The model under review builds one solid part; all positions refer to its coordinate system, in mm. A direction names the side the tool comes from. Coordinates: 2 decimals unless noted, no trailing zeros. Write each loop counter-clockwise with the first axis right and the second up, starting at its lowest first coordinate (ties: lowest second). Pieces come first, ordered by that corner, then holes. Notation, with made-up numbers: (5, -39.5) - (32, -39.5) arc R22 cw to (32, -21.5) - close; hole circle Ø8 at (3.5, 67.25). An arc over 180 degrees is marked (long way). Return JSON: item names as keys, results as strings. Group by question number.
(1) We need section D-D on x = -22.5. State the section outline as (y, z) points, then the cut area to 3 significant figures.
(2) To check wall thickness, follow L1, parallel to X at y = 18.75, z = 26; L2, parallel to Z at x = -27, y = 4; L3, parallel to Y at x = 6, z = 4.5. State the ranges of each line that lie inside material, in increasing order. Write a range as from..to.
(3) We need section B-B on z = -10. State the section outline as (x, y) points, then the cut area to 3 significant figures.
(4) We need section C-C on y = 5. State the section outline as (x, z) points.
(5) We need section A-A on y = 28.25. State the section outline as (x, z) points.
(6) For pin 1 Ø1.5 at (x, y) = (-38.5, 9) entering from +Z; pin 2 Ø3 at (x, z) = (19, 0) entering from +Y; pin 3 Ø1.5 at (x, y) = (-39, 7.5) entering from +Z, all flat-tipped, find the tip position at first contact; note any pin that passes through.
(7) Tool access review of faces 1 (the face through (-38.498, 12.077, -5.534)), 2 (the face through (-4, 16, -25.555)), 3 (the face through (-39.122, 14.79, -27.653)): name each direction out of +Z, -Z, +X, -X, +Y, -Y from which nothing blocks a thin tool from reaching the whole face with its end or side.
(8) Draft analysis for pull direction X (two halves, no side actions). For faces 4 (the face through (-39.977, 15, 12)), 5 (the face through (-38, 13.596, -10)), 6 (the face through (-36.38, 15.7, 47.87)), state which applies: released by +X, released by -X, zero draft, split by the parting line, or undercut.
```python
from build123d import *

# Parameters (mm, degrees)
BOSS_EXTRUDE1_DEPTH = 30
CUT_EXTRUDE1_DEPTH  = 29
CUT_EXTRUDE3_DEPTH  = 10
SKETCH6_W           = 27.115913197
SKETCH6_H           = 16.602687323
BOSS_EXTRUDE2_DEPTH = 3
SKETCH7_W           = 8.89
SKETCH7_H           = 10.922
CUT_EXTRUDE4_DEPTH  = 6350
BOSS_EXTRUDE3_START = -3
SKETCH8_W           = 8.89
SKETCH8_H           = 10.922
BOSS_EXTRUDE3_DEPTH = 3
BOSS_EXTRUDE4_START = -3
SKETCH9_W           = 8.89
SKETCH9_H           = 10.922
BOSS_EXTRUDE4_DEPTH = 3
SKETCH12_W          = 9
SKETCH12_H          = 11
CUT_EXTRUDE6_DEPTH  = 3


with BuildPart() as part:
    # Sketch2 → Boss-Extrude1 (new body)
    with BuildSketch(Plane(origin=(0, 0, 0), x_dir=(1, 0, 0), z_dir=(0, 1, 0))):
        with BuildLine():
            Line((-36.97733711, 28.555240793), (29.02266289, 28.555240793))
            ThreePointArc((29.02266289, 28.555240793), (31.143983233, 27.676561137), (32.02266289, 25.555240793))
            Line((32.02266289, 25.555240793), (32.02266289, -48.444759207))
            ThreePointArc((32.02266289, -48.444759207), (31.143983233, -50.56607955), (29.02266289, -51.444759207))
            Line((29.02266289, -51.444759207), (-36.97733711, -51.444759207))
            ThreePointArc((-36.97733711, -51.444759207), (-39.098657454, -50.56607955), (-39.97733711, -48.444759207))
            Line((-39.97733711, -48.444759207), (-39.97733711, 25.555240793))
            ThreePointArc((-39.97733711, 25.555240793), (-39.098657454, 27.676561137), (-36.97733711, 28.555240793))
        make_face()
    extrude(amount=BOSS_EXTRUDE1_DEPTH)

    # Sketch3 → Cut-Extrude1 (cut)
    with BuildSketch(Plane(origin=(0, 30, 0), x_dir=(1, 0, 0), z_dir=(0, 1, 0))):
        with BuildLine():
            Line((-34.97733711, 25.555240793), (27.02266289, 25.555240793))
            ThreePointArc((27.02266289, 25.555240793), (28.436876452, 24.969454356), (29.02266289, 23.555240793))
            Line((29.02266289, 23.555240793), (29.02266289, -46.444759207))
            ThreePointArc((29.02266289, -46.444759207), (28.436876452, -47.858972769), (27.02266289, -48.444759207))
            Line((27.02266289, -48.444759207), (-34.97733711, -48.444759207))
            ThreePointArc((-34.97733711, -48.444759207), (-36.391550673, -47.858972769), (-36.97733711, -46.444759207))
            Line((-36.97733711, -46.444759207), (-36.97733711, 23.555240793))
            ThreePointArc((-36.97733711, 23.555240793), (-36.391550673, 24.969454356), (-34.97733711, 25.555240793))
        make_face()
    extrude(amount=-CUT_EXTRUDE1_DEPTH, mode=Mode.SUBTRACT)

    # Sketch5 → Cut-Extrude3 (cut)
    with BuildSketch(Plane.ZY.offset(39.97733711)):
        Polygon((14.109885792, 14.391226726), (9.109885792, 14.391226726), (6.109885792, 11.394962385), (6.109885792, 2.391226726), (17.109885792, 2.391226726), (17.109885792, 11.394962385), align=None)
    extrude(amount=-CUT_EXTRUDE3_DEPTH, mode=Mode.SUBTRACT)

    # Sketch6 → Boss-Extrude2 (add)
    with BuildSketch(Plane.ZY.offset(39.97733711)):
        with Locations((11.822368645, 9.478185332)):
            Rectangle(SKETCH6_W, SKETCH6_H)
    extrude(amount=-BOSS_EXTRUDE2_DEPTH)

    # Sketch7 → Cut-Extrude4 (cut)
    with BuildSketch(Plane.XY.offset(51.444759207)):
        Polygon((-29.154490055, 10.403434977), (-26.106490055, 13.462), (-20.275055078, 13.462), (-17.216490055, 10.414), (-17.216490055, 2.54), (-29.154490055, 2.54), align=None)
        with Locations((19.417783934, 8.001)):
            Rectangle(SKETCH7_W, SKETCH7_H)
    extrude(amount=-CUT_EXTRUDE4_DEPTH, mode=Mode.SUBTRACT)

    # Sketch8 → Boss-Extrude3 (add)
    with BuildSketch(Plane(origin=(0, 0, -28.555240793), x_dir=(-1, 0, 0), z_dir=(0, 0, -1)).offset(BOSS_EXTRUDE3_START)):
        Polygon((26.106490055, 13.462), (20.275055078, 13.462), (17.216490055, 10.414), (17.216490055, 2.54), (29.154490055, 2.54), (29.154490055, 10.403434977), align=None)
        with Locations((-19.417783934, 8.001)):
            Rectangle(SKETCH8_W, SKETCH8_H)
    extrude(amount=BOSS_EXTRUDE3_DEPTH)

    # Sketch9 → Boss-Extrude4 (add)
    with BuildSketch(Plane.XY.offset(51.444759207).offset(BOSS_EXTRUDE4_START)):
        Polygon((-29.154490055, 2.54), (-17.216490055, 2.54), (-17.216490055, 10.414), (-20.275055078, 13.462), (-26.106490055, 13.462), (-29.154490055, 10.403434977), align=None)
        with Locations((19.417783934, 8.001)):
            Rectangle(SKETCH9_W, SKETCH9_H)
    extrude(amount=BOSS_EXTRUDE4_DEPTH)

    # Sketch12 → Cut-Extrude6 (cut)
    with BuildSketch(Plane.ZY.offset(39.97733711)):
        Polygon((-16.055240793, 10.6), (-16.055240793, 2.6), (-4.055240793, 2.6), (-4.055240793, 10.6), (-7.055240793, 13.596264341), (-13.055240793, 13.596264341), align=None)
        with Locations((16.944759207, 8.1)):
            Rectangle(SKETCH12_W, SKETCH12_H)
    extrude(amount=-CUT_EXTRUDE6_DEPTH, mode=Mode.SUBTRACT)


solid = part.part
```
Ans:
{
 "1": {"outline": "(0, -28.56) - (30, -28.56) - (30, -25.56) - (1, -25.56) - (1, 48.44) - (30, 48.44) - (30, 51.44) - (0, 51.44) - close", "area": "254 mm²"},
 "2": {"L1": "-39.98..-36.98, 29.02..32.02", "L2": "-28.56..-25.56, 48.44..51.44", "L3": "0..1"},
 "3": {"outline": "(-39.98, 0) - (32.02, 0) - (32.02, 30) - (29.02, 30) - (29.02, 1) - (-36.98, 1) - (-36.98, 2.6) - (-39.98, 2.6) - close; (-39.98, 13.6) - (-36.98, 13.6) - (-36.98, 30) - (-39.98, 30) - close", "area": "213 mm²"},
 "4": {"outline": "(-39.98, -25.56) arc R3 ccw to (-36.98, -28.56) - (29.02, -28.56) arc R3 ccw to (32.02, -25.56) - (32.02, 48.44) arc R3 ccw to (29.02, 51.44) - (-36.98, 51.44) arc R3 ccw to (-39.98, 48.44) - (-39.98, 21.44) - (-36.98, 21.44) - (-36.98, 46.44) arc R2 cw to (-34.98, 48.44) - (27.02, 48.44) arc R2 cw to (29.02, 46.44) - (29.02, -23.56) arc R2 cw to (27.02, -25.56) - (-34.98, -25.56) arc R2 cw to (-36.98, -23.56) - (-36.98, -16.06) - (-39.98, -16.06) - close; (-39.98, -4.06) - (-36.98, -4.06) - (-36.98, 12.44) - (-39.98, 12.44) - close"},
 "5": {"outline": "(-39.98, -25.56) arc R3 ccw to (-36.98, -28.56) - (29.02, -28.56) arc R3 ccw to (32.02, -25.56) - (32.02, 48.44) arc R3 ccw to (29.02, 51.44) - (-36.98, 51.44) arc R3 ccw to (-39.98, 48.44) - close; hole (-36.98, -23.56) arc R2 ccw to (-34.98, -25.56) - (27.02, -25.56) arc R2 ccw to (29.02, -23.56) - (29.02, 46.44) arc R2 ccw to (27.02, 48.44) - (-34.98, 48.44) arc R2 ccw to (-36.98, 46.44) - close"},
 "6": {"pin 1": "z = 51.34", "pin 2": "y = 1", "pin 3": "z = 51.16"},
 "7": {"face 1": "-X", "face 2": "+Y", "face 3": "-Z, -X, +Y, -Y"},
 "8": {"face 4": "released by -X", "face 5": "zero draft", "face 6": "undercut"}
}
